```python
from build123d import *

# Parameters (mm, degrees)
SKETCH1_W           = 125
SKETCH1_H           = 140
BOSS_EXTRUDE1_DEPTH = 3.18
SKETCH2_R           = 1.5
SKETCH2_W           = 3.18
SKETCH2_H           = 60.125
CUT_EXTRUDE1_DEPTH  = 4.18
CUT_EXTRUDE5_DEPTH  = 12
SKETCH5_R           = 32.671394307
CUT_EXTRUDE6_DEPTH  = 10
SKETCH9_R           = 1.042012373
CUT_EXTRUDE8_DEPTH  = 4.18


with BuildPart() as part:
    # Sketch1 → Boss-Extrude1 (new body)
    with BuildSketch(Plane.XY):
        Rectangle(SKETCH1_W, SKETCH1_H)
    extrude(amount=BOSS_EXTRUDE1_DEPTH)

    # Sketch2 → Cut-Extrude1 (cut, through all)
    with BuildSketch(Plane.XY.offset(3.18)):
        with Locations((-60.5, 0)):
            Circle(SKETCH2_R)
        with Locations((60.5, 0)):
            Circle(SKETCH2_R)
        Polygon((-10, 70), (10, 70), (10, 66.82), (1.5, 66.82), (1.5, 62.82), (3.5, 62.82), (3.5, 59.82), (1.5, 59.82), (1.5, 56.82), (-1.5, 56.82), (-1.5, 59.82), (-3.5, 59.82), (-3.5, 62.82), (-1.5, 62.82), (-1.5, 66.82), (-10, 66.82), align=None)
        Polygon((-10, -70), (-10, -66.82), (-1.5, -66.82), (-1.5, -62.82), (-3.5, -62.82), (-3.5, -59.82), (-1.5, -59.82), (-1.5, -56.82), (1.5, -56.82), (1.5, -59.82), (3.5, -59.82), (3.5, -62.82), (1.5, -62.82), (1.5, -66.82), (10, -66.82), (10, -70), align=None)
        with Locations((-60.91, 39.9375)):
            Rectangle(SKETCH2_W, SKETCH2_H)
        with Locations((-60.91, -39.9375)):
            Rectangle(SKETCH2_W, SKETCH2_H)
        with Locations((60.91, -39.9375)):
            Rectangle(SKETCH2_W, SKETCH2_H)
        with Locations((60.91, 39.9375)):
            Rectangle(SKETCH2_W, SKETCH2_H)
    extrude(amount=-CUT_EXTRUDE1_DEPTH, mode=Mode.SUBTRACT)

    # Sketch4 → Cut-Extrude5 (cut)
    with BuildSketch(Plane.XY):
        with BuildLine():
            Line((-25.57107609, -41.8625), (-45.57107609, -41.8625))
            Line((-45.57107609, -41.8625), (-45.57107609, -45.3625))
            Line((-45.57107609, -45.3625), (-48.57107609, -45.3625))
            Line((-48.57107609, -45.3625), (-48.57107609, -34.3625))
            Line((-48.57107609, -34.3625), (-45.57107609, -34.3625))
            Line((-45.57107609, -34.3625), (-45.57107609, -37.8625))
            Line((-45.57107609, -37.8625), (-31.57107609, -37.8625))
            Line((-31.57107609, -37.8625), (-31.57107609, -33.087601989))
            Line((-31.57107609, -33.087601989), (-28.57107609, -33.087601989))
            ThreePointArc((-28.57107609, -33.087601989), (-27.787526444, -36.79230316), (-25.57107609, -39.8625))
            Line((-25.57107609, -39.8625), (-25.57107609, -41.8625))
        make_face()
    extrude(amount=CUT_EXTRUDE5_DEPTH, mode=Mode.SUBTRACT)

    # Sketch5 → Cut-Extrude6 (cut)
    with BuildSketch(Plane.XY.offset(3.18)):
        with Locations((11.462576996, 0)):
            Circle(SKETCH5_R)
    extrude(amount=-CUT_EXTRUDE6_DEPTH, mode=Mode.SUBTRACT)

    # Sketch9 → Cut-Extrude8 (cut, through all)
    with BuildSketch(Plane.XY.offset(3.18)):
        with Locations((37.991387583, -21.1)):
            Circle(SKETCH9_R)
        with Locations((37.991387583, 21.008299604)):
            Circle(SKETCH9_R)
    extrude(amount=-CUT_EXTRUDE8_DEPTH, mode=Mode.SUBTRACT)


solid = part.part
```
Read the model definition and answer for the solid it produces. Units are mm, in the model's axes. A direction names the side the tool comes from. Give positions to 0.01 mm unless a question says otherwise; leave off trailing zeros. Write each loop counter-clockwise with the first axis right and the second up, starting at its lowest first coordinate (ties: lowest second). Pieces come first, ordered by that corner, then holes. Notation, with made-up numbers: (44.5, 66) - (101.5, 66) arc R10 cw to (101.5, 76) - close; hole circle Ø5 at (85, -26.5). An arc over 180 degrees is marked (long way). Write item = value, one per line. Start each with the question number.
Item 1: Find section C-C (y = -50). Give the vertices of the cut face in (x, z), then the cut area to 3 significant figures.
Item 2: Find section D-D (z = 1.35). State how many separate pieces and enclosed holes the cut face has, then the cut area to 3 significant figures.
Item 3: Each of these flat-tipped pins is pushed along its axis until it touches: P1, Ø1.6, axis at y = -40.5, z = 2.5, coming from the -X side; P2, Ø3.5, axis at x = 37.99, y = -21.1, coming from the -Z side; P3, Ø0.6, axis at x = 2, z = 1.5, coming from the -Y side; P4, Ø1, axis at x = 2.5, z = 2, coming from the +Y side. Where does it stop, or does it pass through?
Item 4: Find section A-A (x = 7). Give the vertices of the cut face in (y, z).
Item 5: Find the intervals of material crossed by probe 1 along Y at (x, z) = (-30.5, 2.4); probe 2 along Y at (x, z) = (-43, 0.5); probe 3 along X at (y, z) = (-42.5, 0.35), in increasing order. Write a range as [from, to].
Item 6: A tool of negligible diameter and unlimited length cuts with its end or side. For faces 5 (the flat face through (-47, -34.362, 2)), 6 (the flat face through (1.5, 58, 2)), 7 (the flat face through (-1.5, -65, 2)), from which of +Z, -Z, +X, -X, +Y, -Y can it reach the whole face along a straight path? Write none if from no direction.
Item 7: Find section B-B (y = -4). Give the vertices of the cut face in (x, z).
Item 8: The mould has two halves that part along Y. Classify faces 1 (the flat face through (-6, -66.82, 2)), 2 (the flat face through (-47, -45.362, 2)), 3 (the flat face through (59.32, -40, 2)), 4 (the flat face through (-35, 70, 2)): +Y half, -Y half, draft (parallel to the pull), parting line (faces both ways), or undercut.
Response:
q1.outline = (-59.32, 0) - (59.32, 0) - (59.32, 3.18) - (-59.32, 3.18) - close
q1.area = 377 mm²
q2.separate_pieces = 1
q2.enclosed_holes = 6
q2.area = 13,000 mm²
q3.P1 = -59.32
q3.P2 = 0
q3.P3 = -66.82
q3.P4 = 66.82
q4.outline = (-66.82, 0) - (-32.37, 0) - (-32.37, 3.18) - (-66.82, 3.18) - close; (32.37, 0) - (66.82, 0) - (66.82, 3.18) - (32.37, 3.18) - close
q5.probe_1 = [-70, -41.86], [-33.09, 70]
q5.probe_2 = [-70, -41.86], [-37.86, 70]
q5.probe_3 = [-59.32, -48.57], [-45.57, 59.32]
q6.face_5 = +Z, -Z
q6.face_6 = +Z, -Z, +Y
q6.face_7 = +Z, -Z, -Y
q7.outline = (-62.5, 0) - (-20.96, 0) - (-20.96, 3.18) - (-62.5, 3.18) - close; (43.89, 0) - (62.5, 0) - (62.5, 3.18) - (43.89, 3.18) - close
q8.face_1 = -Y half
q8.face_2 = undercut
q8.face_3 = draft
q8.face_4 = +Y half
